```python
from build123d import *

# Parameters (mm, degrees)
SKETCH1_W           = 62
SKETCH1_H           = 8
BOSS_EXTRUDE1_DEPTH = 5
SKETCH2_R           = 1.5
CUT_EXTRUDE1_DEPTH  = 10


with BuildPart() as part:
    # Sketch1 → Boss-Extrude1 (new body)
    with BuildSketch(Plane.XY):
        Rectangle(SKETCH1_W, SKETCH1_H)
    extrude(amount=BOSS_EXTRUDE1_DEPTH)

    # Sketch2 → Cut-Extrude1 (cut)
    with BuildSketch(Plane(origin=(0, 0, 0), x_dir=(-1, 0, 0), z_dir=(0, 0, -1))):
        with Locations((-25, 0)):
            Circle(SKETCH2_R)
        Circle(SKETCH2_R)
        with Locations((25, 0)):
            Circle(SKETCH2_R)
    extrude(amount=-CUT_EXTRUDE1_DEPTH, mode=Mode.SUBTRACT)


solid = part.part
```
The listing builds one solid part. Answer for the finished solid, in the listing's coordinates (mm). Give positions to 0.01 mm unless a question says otherwise; leave off trailing zeros. Order: outer loops, then holes, each group sorted by start corner. A loop starts at its lowest first (then second) coordinate and runs counter-clockwise, first axis right, second up. Notation, with made-up numbers: (76.25, 17.5) - (122.25, 17.5) arc R13 ccw to (122.25, 29.5) - close; hole circle Ø5 at (33, 7). An arc over 180 degrees is marked (long way). Use one line per item in the form item = value. Start each with the question number.
(1) The mould has two halves that part along Y. Classify faces 1 (the cylindrical face through (1.5, 0.07, 2.46)), 2 (the flat face through (0, -4, 2)), 3 (the flat face through (0, 4, 2)), 4 (the cylindrical face through (-23.5, 0.07, 2.46)): released by +Y, released by -Y, zero draft, split by the parting line, or undercut.
(2) Flat-ended cylindrical pins translate along their axes: pin 1 Ø1.8 at (x, y) = (25, 0) entering from +Z; pin 2 Ø4 at (x, y) = (-25, 0) entering from +Z. Find the tip coordinate at first contact, or state that the pin passes through.
(3) A cutting plane is placed at B-B, the plane y = 0. Write down the section's boundary in (x, z).
(4) Consider line 1 (Y direction, x = -25, z = 1.7); line 2 (X direction, y = 0.75, z = 0.55). Determine where each line is inside the solid, lowest interval first. Write a range as from..to.
(5) A cutting plane is placed at A-A, the plane x = 25. Write down the section's boundary in (y, z), then the cut area to 3 significant figures.
(6) A cutting plane is placed at C-C, the plane z = 3.1. Write down the section's boundary in (x, y), then the cut area to 3 significant figures.
Ans:
q1.face_1 = undercut
q1.face_2 = released by -Y
q1.face_3 = released by +Y
q1.face_4 = undercut
q2.pin_1 = through
q2.pin_2 = 5
q3.outline = (-31, 0) - (-26.5, 0) - (-26.5, 5) - (-31, 5) - close; (-23.5, 0) - (-1.5, 0) - (-1.5, 5) - (-23.5, 5) - close; (1.5, 0) - (23.5, 0) - (23.5, 5) - (1.5, 5) - close; (26.5, 0) - (31, 0) - (31, 5) - (26.5, 5) - close
q4.line_1 = -4..-1.5, 1.5..4
q4.line_2 = -31..-26.3, -23.7..-1.3, 1.3..23.7, 26.3..31
q5.outline = (-4, 0) - (-1.5, 0) - (-1.5, 5) - (-4, 5) - close; (1.5, 0) - (4, 0) - (4, 5) - (1.5, 5) - close
q5.area = 25.0 mm^2
q6.outline = (-31, -4) - (31, -4) - (31, 4) - (-31, 4) - close; hole circle Ø3 at (-25, 0); hole circle Ø3 at (0, 0); hole circle Ø3 at (25, 0)
q6.area = 475 mm^2
